Model file for the job. Use its own axes, mm. A direction names the side the tool comes from. Coordinates: 2 decimals unless noted, no trailing zeros. Write each loop counter-clockwise with the first axis right and the second up, starting at its lowest first coordinate (ties: lowest second). Pieces come first, ordered by that corner, then holes. Notation, with made-up numbers: M 71,-2 L 83,-2 A11 ccw 83,13 Z; hole C 11,24 d3. An arc over 180 degrees is marked long. Put each result on its own line as item: value. Start each with the question number.
Q1. Drill centre lines: line 1 along Z through (x, y) = (11.5, -7.25); line 2 along Y through (x, z) = (7.5, -24); line 3 along Z through (x, y) = (0.75, 11.5). Where is each one in solid material? Low to high.
Q2. Which spindle directions (+Z, -Z, +X, -X, +Y, -Y) get a long thin tool onto all of the face, cutting with end or side? Do faces 1 (the flat face through (0.1, 10.2, -25)), 2 (the flat face through (2.2, 12.5, 12)), 3 (the flat face through (0, -13, 0)). Say none if no direction does.
Q3. Drop flat-ended pins along their axis: pin 1 (8 mm diameter, centred on x = -6, z = -19.5, fed in from +Y); pin 2 (5 mm diameter, centred on x = -12, y = 2, fed in from -Z); pin 3 (1 mm diameter, centred on x = -6.5, y = 11.5, fed in from -Z). Give the stop position or say it passes through.
Q4. Cut at C-C (z = 6). Write the cut outline in (x, y).
Q5. Cut at B-B (y = 0). Write the cut outline in (x, z), then the cut area to 3 significant figures.
Q6. Cut at A-A (x = 0). Write the cut outline in (y, z), then the cut area to 3 significant figures.
```python
from build123d import *

# Parameters (mm, degrees)
F3_DEPTH      = 25
F3_DEPTH_BACK = 25
F4_SIZE       = 1


with BuildPart() as f1:
    # F0 (on Front) → F1 (revolve)
    with BuildSketch(Plane.XZ):
        Polygon((-12.5, 12), (-15, 12), (-15, 0), (-15, -12), (-12.5, -12), (-12.5, -25), (-10, -25), (-10, -70), (0, -70), (0, 0), (0, 70), (-10, 70), (-10, 25), (-12.5, 25), align=None)
    revolve(axis=Axis((0, 0, 35), (0, 0, -1)))

    # F2 (on Top) → F3 (cut, two sides)
    with BuildSketch(Plane.XY) as f3_sk:
        Polygon((0, -13), (-15, -13), (-15, -17), (0, -17), (15, -17), (15, -13), align=None)
    extrude(amount=F3_DEPTH, mode=Mode.SUBTRACT)
    extrude(f3_sk.sketch, amount=-F3_DEPTH_BACK, mode=Mode.SUBTRACT)

    # F4
    f4_edges = [f1.edges().sort_by_distance(p)[0] for p in [
        (10, 0, 70),
        (10, 0, -70),
    ]]
    chamfer(f4_edges, length=F4_SIZE)


solid = f1.part
```
Computed values:
1. line 1: -12 to 12
1. line 2: -10 to 10
1. line 3: -25 to 25
2. face 1: -Z
2. face 2: +Z
2. face 3: +Z, -Z, +X, -X, -Y
3. pin 1: y = 12.34
3. pin 2: z = -69.33
3. pin 3: z = -12
4. outline: M -7.48,-13 L 7.48,-13 A15 ccw long Z
5. outline: M -15,-12 L -12.5,-12 L -12.5,-25 L -10,-25 L -10,-69 L -9,-70 L 9,-70 L 10,-69 L 10,-25 L 12.5,-25 L 12.5,-12 L 15,-12 L 15,12 L 12.5,12 L 12.5,25 L 10,25 L 10,69 L 9,70 L -9,70 L -10,69 L -10,25 L -12.5,25 L -12.5,12 L -15,12 Z
5. area: 3,170 mm2
6. outline: M -13,-12 L -12.5,-12 L -12.5,-25 L -10,-25 L -10,-69 L -9,-70 L 9,-70 L 10,-69 L 10,-25 L 12.5,-25 L 12.5,-12 L 15,-12 L 15,12 L 12.5,12 L 12.5,25 L 10,25 L 10,69 L 9,70 L -9,70 L -10,69 L -10,25 L -12.5,25 L -12.5,12 L -13,12 Z
6. area: 3,120 mm2
